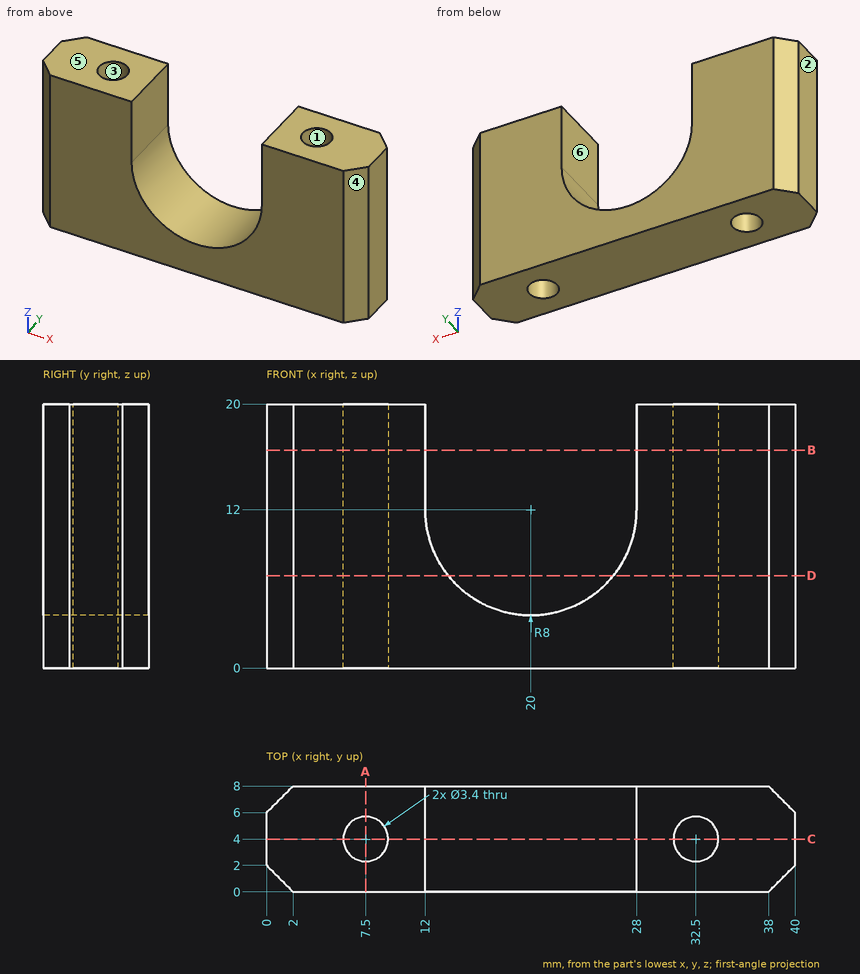
Geometry: see drawing. Coordinates: mm, zero at the bounding-box minimum. A direction names the side the tool comes from. Coordinates: 2 decimals unless noted, no trailing zeros. Order: outer loops, then holes, each group sorted by start corner. A loop starts at its lowest first (then second) coordinate and runs counter-clockwise, first axis right, second up. Notation, with made-up numbers: M 4.25,-7.5 L 45.25,-7.5 A7 ccw 45.25,3.5 Z; hole C -25.5,-17.5 d5. An arc over 180 degrees is marked long. Write item = value, one per line. Start each with the question number.
(1) First-contact query: P1, Ø2, axis at x = 7.5, y = 4, coming from the +Z side. Flat tip, straight axial feed; report the tip coordinate or a pass-through.
(2) Section C-C on y = 4. Output: boundary loops of the cut face in (x, z).
(3) Section A-A on x = 7.5. Output: boundary loops of the cut face in (y, z).
(4) Line query: line 1 along Y through (x, z) = (7.5, 10.5); line 2 along X through (y, z) = (4.5, 2); line 3 along X through (y, z) = (1.5, 18.75). Output: solid intervals per line, ascending. Write a range as [from, to].
(5) Section D-D on z = 7. Output: boundary loops of the cut face in (x, y) (3 decimals), and give its area (3 significant figures).
(6) Section B-B on z = 16.5. Output: boundary loops of the cut face in (x, y).
(7) Reachability of the marked faces 5 and 6 from +Z, -Z, +X, -X, +Y, -Y: full face, straight path, thin tool, end or side. Return the list, or none.
(8) Pull-direction query (Y, two-part tool) for the marked faces 1, 2, 3 and 4; classes: released by +Y, released by -Y, zero draft, split by the parting line, or undercut.
Result set:
q1.P1 = through
q2.outline = M 0,0 L 5.8,0 L 5.8,20 L 0,20 Z; M 9.2,0 L 30.8,0 L 30.8,20 L 28,20 L 28,12 A8 cw 12,12 L 12,20 L 9.2,20 Z; M 34.2,0 L 40,0 L 40,20 L 34.2,20 Z
q3.outline = M 0,0 L 2.3,0 L 2.3,20 L 0,20 Z; M 5.7,0 L 8,0 L 8,20 L 5.7,20 Z
q4.line_1 = [0, 2.3], [5.7, 8]
q4.line_2 = [0, 5.88], [9.12, 30.88], [34.12, 40]
q4.line_3 = [0.5, 12], [28, 39.5]
q5.outline = M 0,2 L 2,0 L 13.755,0 L 13.755,8 L 2,8 L 0,6 Z; M 26.245,0 L 38,0 L 40,2 L 40,6 L 38,8 L 26.245,8 Z; hole C 7.5,4 d3.4; hole C 32.5,4 d3.4
q5.area = 194 mm²
q6.outline = M 0,2 L 2,0 L 12,0 L 12,8 L 2,8 L 0,6 Z; M 28,0 L 38,0 L 40,2 L 40,6 L 38,8 L 28,8 Z; hole C 7.5,4 d3.4; hole C 32.5,4 d3.4
q7.face_5 = +Z, +X, -X, +Y, -Y
q7.face_6 = +Z, +Y, -Y
q8.face_1 = undercut
q8.face_2 = zero draft
q8.face_3 = undercut
q8.face_4 = released by -Y
